```python
from build123d import *

# Parameters (mm, degrees)
SKETCH_1_R      = 31.5
EXTRUDE_1_DEPTH = 2
SKETCH_2_R      = 31.5
SKETCH_2_R_2    = 30
EXTRUDE_2_DEPTH = 1.3
EXTRUDE_START   = 1.3
SKETCH_3_R      = 31.5
SKETCH_3_R_2    = 30
EXTRUDE_3_DEPTH = 1.3


with BuildPart() as part:
    # 스케치1 → 보스-돌출1 (new body)
    with BuildSketch(Plane.XY):
        Circle(SKETCH_1_R)
    extrude(amount=EXTRUDE_1_DEPTH)

    # 스케치2 → 보스-돌출2 (add)
    with BuildSketch(Plane.XY.offset(2)):
        Circle(SKETCH_2_R)
        Circle(SKETCH_2_R_2, mode=Mode.SUBTRACT)
    extrude(amount=EXTRUDE_2_DEPTH)

    # 스케치3 → 보스-돌출3 (add)
    with BuildSketch(Plane(origin=(0, 0, 0), x_dir=(-1, 0, 0), z_dir=(0, 0, -1)).offset(EXTRUDE_START)):
        Circle(SKETCH_3_R)
        with Locations(Location((0, 0, 0), (0, 0, 180))):
            Circle(SKETCH_3_R_2, mode=Mode.SUBTRACT)
    extrude(amount=-EXTRUDE_3_DEPTH)


solid = part.part
```
Geometry check sheet. Reference: the model listing, model coordinates, mm. A direction names the side the tool comes from. Give positions to 0.01 mm unless a question says otherwise; leave off trailing zeros. Loops run counter-clockwise (first coordinate to the right, second up) from the corner with the lowest first, then second, coordinate; pieces in that order, holes last. Notation, with made-up numbers: (38, -13.75) - (64, -13.75) arc R23 ccw to (64, -4.75) - close; hole circle Ø7 at (60, -3.5). An arc over 180 degrees is marked (long way). Use CSV: the item, a comma, the result in double quotes. Start each with the question number.
Q1. Release check for a two-part mould opening along X. For faces 1 (the face through (-28, -12, -1.3)), 2 (the face through (0, 0, 2)), 3 (the face through (16.128, -25.296, -0.659)) record: +X half, -X half, draft (parallel to the pull), parting line (faces both ways), or undercut.
Q2. Go/stop test with flat-tipped pins: pin 1 Ø1.5 at (x, y) = (16.5, 12.5) entering from +Z; pin 2 Ø5 at (x, y) = (-7.5, 6.5) entering from -Z; pin 3 Ø1 at (y, z) = (-14.5, -1) entering from +X. Record where each tip stops, or that it passes through.
Q3. Access from +Z, -Z, +X, -X, +Y, -Y to the whole of each face (thin tool, end or side, straight path). Record for faces 4 (the face through (-29.97, 1.32, 2.64)), 5 (the face through (0, 0, 0)), 6 (the face through (28, -12, 3.3)).
Q4. Section check A-A, the plane x = 0. Record the cut outline in (y, z).
Q5. Scan lines: probe 1 along Y at (x, z) = (0, 2.9); probe 2 along Z at (x, y) = (0, -5); probe 3 along X at (y, z) = (-15, 3). Record each from-to range of solid material in increasing order. Write a range as from..to.
Findings below:
1,face 1,"draft"
1,face 2,"undercut"
1,face 3,"undercut"
2,pin 1,"stops at z = 2"
2,pin 2,"stops at z = 0"
2,pin 3,"stops at x = 28.22"
3,face 4,"+Z"
3,face 5,"-Z"
3,face 6,"+Z, +X, -X, +Y, -Y"
4,outline,"(-31.5, -1.3) - (-30, -1.3) - (-30, 0) - (30, 0) - (30, -1.3) - (31.5, -1.3) - (31.5, 3.3) - (30, 3.3) - (30, 2) - (-30, 2) - (-30, 3.3) - (-31.5, 3.3) - close"
5,probe 1,"y = -31.5..-30, 30..31.5"
5,probe 2,"z = 0..2"
5,probe 3,"x = -27.7..-25.98, 25.98..27.7"
